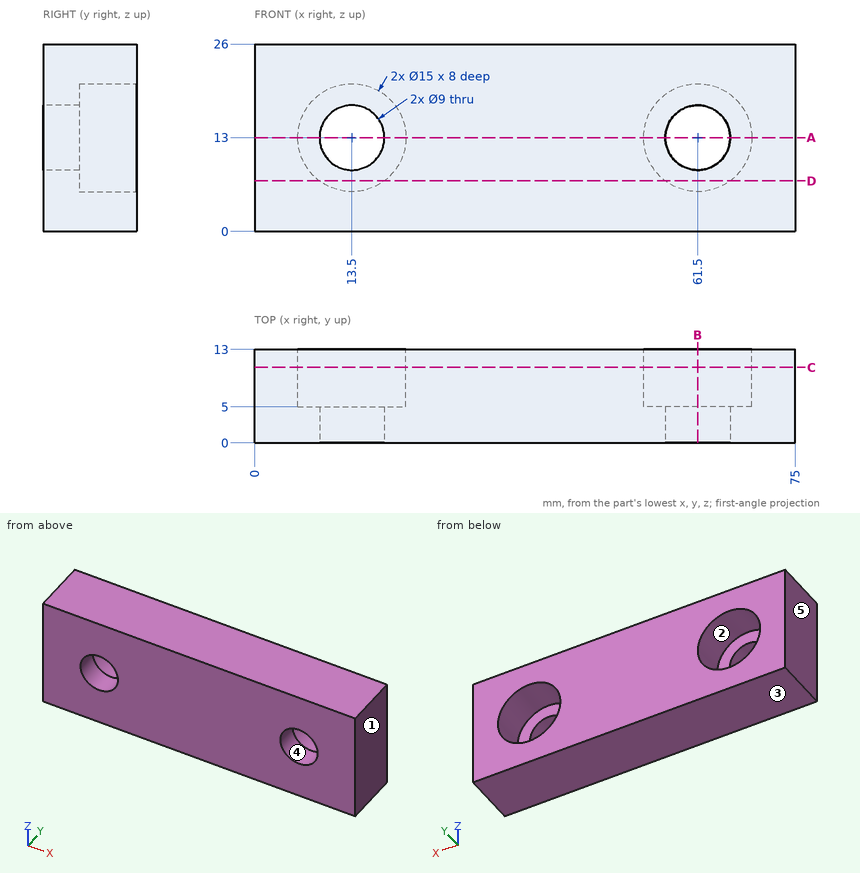
Print and shaded views of the part. All mm, measured from the part's lowest x, y and z. A direction names the side the tool comes from. Round coordinates to 2 decimals unless told otherwise and drop trailing zeros. Write each loop counter-clockwise with the first axis right and the second up, starting at its lowest first coordinate (ties: lowest second). Pieces come first, ordered by that corner, then holes. Notation, with made-up numbers: M 39,-6 L 89,-6 A28 cw 89,29 Z; hole C -37,71.5 d1. An arc over 180 degrees is marked long. Use a Markdown table: item, result. Add a question column.
1. Slice it at C-C on y = 10.5. Give the cut face in (x, z).
2. Flat gauge pins, fed straight in: P1, Ø8, axis at x = 61.5, z = 13, coming from the -Y side; P2, Ø7.5, axis at x = 58.5, z = 12.5, coming from the +Y side. Where does each tip first touch, or does it go through?
3. Drill centre lines: probe 1 along Z at (x, y) = (13.5, 9); probe 2 along X at (y, z) = (7.25, 7.25); probe 3 along Z at (x, y) = (19.5, 12). Where is each one in solid material? Low to high.
4. Slice it at D-D on z = 7. Give the cut face in (x, y), then the cut area to 3 significant figures.
5. Pull direction X, two halves, no side cores. Call the marked faces 3, 4 and 5: released by +X, released by -X, zero draft, split by the parting line, or undercut.
6. 3-axis set-ups, long thin cutter, end or side, ignore diameter. For the marked faces 1 and 2: which of +Z, -Z, +X, -X, +Y, -Y reach the whole face in a straight line?
7. Slice it at A-A on z = 13. Give the cut face in (x, y), then the cut area to 3 significant figures.
8. Slice it at B-B on x = 61.5. Give the cut face in (y, z).
Reply:
| question | item | result |
|---|---|---|
| 1 | outline | M 0,0 L 75,0 L 75,26 L 0,26 Z; hole C 13.5,13 d15; hole C 61.5,13 d15 |
| 2 | P1 | passes through |
| 2 | P2 | stops at y = 5 |
| 3 | probe 1 | z = 0 to 5.5, 20.5 to 26 |
| 3 | probe 2 | x = 0 to 8.68, 18.32 to 56.68, 66.32 to 75 |
| 3 | probe 3 | z = 0 to 8.5, 17.5 to 26 |
| 4 | outline | M 0,0 L 75,0 L 75,13 L 66,13 L 66,5 L 57,5 L 57,13 L 18,13 L 18,5 L 9,5 L 9,13 L 0,13 Z |
| 4 | area | 831 mm^2 |
| 5 | face 3 | zero draft |
| 5 | face 4 | undercut |
| 5 | face 5 | released by -X |
| 6 | face 1 | +Z, -Z, +X, +Y, -Y |
| 6 | face 2 | +Y |
| 7 | outline | M 0,0 L 9,0 L 9,5 L 6,5 L 6,13 L 0,13 Z; M 18,0 L 57,0 L 57,5 L 54,5 L 54,13 L 21,13 L 21,5 L 18,5 Z; M 66,0 L 75,0 L 75,13 L 69,13 L 69,5 L 66,5 Z |
| 7 | area | 645 mm^2 |
| 8 | outline | M 0,0 L 13,0 L 13,5.5 L 5,5.5 L 5,8.5 L 0,8.5 Z; M 0,17.5 L 5,17.5 L 5,20.5 L 13,20.5 L 13,26 L 0,26 Z |
